```python
from build123d import *

# Parameters (mm, degrees)
SKETCH1_R                = 11.25
BOSS_EXTRUDE1_DEPTH      = 2.2
BOSS_EXTRUDE2_DEPTH      = 1.6
BOSS_EXTRUDE2_DEPTH_BACK = 1.6
SKETCH3_W                = 33.32922231
SKETCH3_H                = 16.3
BOSS_EXTRUDE3_DEPTH      = 3.2


with BuildPart() as part:
    # Sketch1 → Boss-Extrude1 (new body)
    with BuildSketch(Plane(origin=(0, 0, 0), x_dir=(1, 0, 0), z_dir=(0, 1, 0))):
        with Locations(Location((0, 0, 0), (0, 0, 270))):
            Circle(SKETCH1_R)
    extrude(amount=BOSS_EXTRUDE1_DEPTH)

    # Sketch2 → Boss-Extrude2 (add, two sides: drawn at the far end of the back side and taken through both)
    with BuildSketch(Plane.XY.offset(-BOSS_EXTRUDE2_DEPTH_BACK)):
        Polygon((-8, 51), (8, 51), (18, 30.5), (18, 20.5), (8, 0), (-8, 0), (-18, 20.5), (-18, 30.5), align=None)
    extrude(amount=BOSS_EXTRUDE2_DEPTH + BOSS_EXTRUDE2_DEPTH_BACK)

    # Sketch3 → Boss-Extrude3 (add)
    with BuildSketch(Plane.XY.offset(1.6)):
        with Locations((29.798803479, 25.5)):
            Rectangle(SKETCH3_W, SKETCH3_H)
    extrude(amount=-BOSS_EXTRUDE3_DEPTH)


solid = part.part
```
Can you work these out from the model? Positions are in its coordinate system, mm. A direction names the side the tool comes from. Give positions to 0.01 mm unless a question says otherwise; leave off trailing zeros. Write each loop counter-clockwise with the first axis right and the second up, starting at its lowest first coordinate (ties: lowest second). Pieces come first, ordered by that corner, then holes. Notation, with made-up numbers: (40.25, -38.5) - (50.25, -38.5) arc R17 cw to (50.25, -11.5) - close; hole circle Ø11 at (31.5, 43). An arc over 180 degrees is marked (long way). Write item = value, one per line. Start each with the question number.
1. Thinking about a two-plate mould opening in Y: for faces 5 (the face through (0, 0, 0)), 6 (the face through (-4.31, 1.08, 10.39)), 7 (the face through (12.82, 9.88, -0.02)), which applies, released by +Y, released by -Y, zero draft, split by the parting line, or undercut?
2. Imagine slicing it at D-D (x = -12). Please give me the cut outline in (y, z), and give its area (3 significant figures).
3. On a 3-axis mill with a long thin cutter (end or side, diameter ignored), from which of +Z, -Z, +X, -X, +Y, -Y can I reach the whole of each face in a straight line? I mean faces 1 (the face through (31, 33.65, 0)), 2 (the face through (8, 27, 1.6)), 3 (the face through (-13.474, 11.222, -0.022)), 4 (the face through (31, 17.35, 0)). Say none if no direction works.
4. Imagine slicing it at A-A (x = 0). Please give me the cut outline in (y, z).
5. For pin 1 (24.5 mm diameter, centred on x = 22.5, y = 37.5, fed in from -Z); pin 2 (2.5 mm diameter, centred on x = 29, z = -0.5, fed in from +Y); pin 3 (4 mm diameter, centred on x = 39.5, y = 31.5, fed in from +Z); pin 4 (10 mm diameter, centred on y = 16, z = -8.5, fed in from +X), each with a flat end and sliding along its axis, tell me the tip position at first contact or that it passes through.
6. Please list where these lines run through material, in increasing order: line 1 (Z direction, x = -8, y = 7); line 2 (Y direction, x = -10, z = -2.75); line 3 (Y direction, x = 31, z = -0.5).
7. Imagine slicing it at B-B (z = 0). Please give me the cut outline in (x, y).
8. Imagine slicing it at C-C (y = 12.5). Please give me the cut outline in (x, z).
Worked answers:
q1.face_5 = released by -Y
q1.face_6 = zero draft
q1.face_7 = undercut
q2.outline = (8.2, -1.6) - (42.8, -1.6) - (42.8, 1.6) - (8.2, 1.6) - close
q2.area = 111 mm2
q3.face_1 = +Z, -Z, +X, +Y
q3.face_2 = +Z, +X, -X, +Y
q3.face_3 = +Z, -Z, -X
q3.face_4 = +Z, -Z, +X, -Y
q4.outline = (0, -11.25) - (2.2, -11.25) - (2.2, -1.6) - (51, -1.6) - (51, 1.6) - (2.2, 1.6) - (2.2, 11.25) - (0, 11.25) - close
q5.pin_1 = -1.6
q5.pin_2 = 33.65
q5.pin_3 = 1.6
q5.pin_4 = through
q6.line_1 = -1.6 to 1.6
q6.line_2 = 0 to 2.2
q6.line_3 = 17.35 to 33.65
q7.outline = (-18, 20.5) - (-9.07, 2.2) - (-11.25, 2.2) - (-11.25, 0) - (11.25, 0) - (11.25, 2.2) - (9.07, 2.2) - (16.46, 17.35) - (46.46, 17.35) - (46.46, 33.65) - (16.46, 33.65) - (8, 51) - (-8, 51) - (-18, 30.5) - close
q8.outline = (-14.1, -1.6) - (14.1, -1.6) - (14.1, 1.6) - (-14.1, 1.6) - close
